Autodesk Inventor part; units mm, degrees
ref_plane "YZ Plane" through (0, 0, 0) normal (1, 0, 0) x (0, 1, 0)
ref_plane "XZ Plane" through (0, 0, 0) normal (0, 1, 0) x (-1, 0, 0)
ref_plane "XY Plane" through (0, 0, 0) normal (0, 0, 1) x (1, 0, 0)
sketch "Sketch1" plane through (0, 0, 0) normal (0, 1, 0) x (-1, 0, 0)
  line L0 (0, 0) -> (0, -140)
  line L1 (0, -140) -> (40, -140)
  line L2 (40, -140) -> (40, 0)
  line L3 (40, 0) -> (0, 0)
  dimension "d0" = 140
  dimension "d1" = 40
extrude "Extrusion1" add sketch "Sketch1" along normal blind 68.5
sketch "Sketch2" plane through (0, 0, 0) normal (1, 0, 0) x (0, 0, -1)
  line L0 (140, 68.5) -> (0, 68.5)
  line L1 (45, 78.5) -> (39, 78.5)
  line L2 (39, 78.5) -> (39, 74.5)
  line L3 (39, 74.5) -> (37.3, 74.5)
  line L4 (37.3, 74.5) -> (37.3, 80.2)
  line L5 (37.3, 80.2) -> (43.5, 80.2)
  line L6 (43.5, 80.2) -> (43.5, 104.7)
  line L7 (43.5, 104.7) -> (37.3, 104.7)
  line L8 (37.3, 104.7) -> (37.3, 110.4)
  line L9 (37.3, 110.4) -> (39, 110.4)
  line L10 (39, 110.4) -> (39, 106.4)
  line L11 (39, 106.4) -> (45, 106.4)
  line L12 (45, 106.4) -> (45, 78.5)
  line L13 (95, 78.5) -> (101, 78.5)
  line L14 (101, 78.5) -> (101, 74.5)
  line L15 (101, 74.5) -> (102.7, 74.5)
  line L16 (102.7, 74.5) -> (102.7, 80.2)
  line L17 (102.7, 80.2) -> (96.5, 80.2)
  line L18 (96.5, 80.2) -> (96.5, 104.7)
  line L19 (96.5, 104.7) -> (102.7, 104.7)
  line L20 (102.7, 104.7) -> (102.7, 110.4)
  line L21 (102.7, 110.4) -> (101, 110.4)
  line L22 (101, 110.4) -> (101, 106.4)
  line L23 (101, 106.4) -> (95, 106.4)
  line L24 (95, 106.4) -> (95, 78.5)
  line L25 (37.3, 68.5) -> (32.3, 68.5)
  line L26 (32.3, 68.5) -> (32.3, 110.4)
  line L27 (32.3, 110.4) -> (32.3, 115.4)
  line L28 (32.3, 115.4) -> (102.7, 115.4)
  line L29 (102.7, 115.4) -> (107.7, 115.4)
  line L30 (107.7, 115.4) -> (107.7, 68.5)
  line L31 (37.3, 68.5) -> (107.7, 68.5)
  point P0 (0, 0)
  dimension "d8" = 4
  dimension "d9" = 1.7
  dimension "d10" = 5.7
  dimension "d11" = 6.2
  dimension "d12" = 24.5
  dimension "d13" = 5.7
  dimension "d14" = 1.7
  dimension "d15" = 4
  dimension "d16" = 6
  dimension "d17" = 5
  dimension "d18" = 5
  dimension "d19" = 5
extrude "Extrusion2" add sketch "Sketch2" against normal up to surface (40 mm away)
sketch "Sketch3" plane through (0, 0, 0) normal (1, 0, 0) x (0, 0, -1)
  line L0 (87.95, 12.7) -> (87.95, 11)
  line L1 (87.95, 11) -> (83.95, 11)
  line L2 (83.95, 11) -> (83.95, 5)
  line L3 (83.95, 5) -> (70, 5)
  line L4 (70, 6.5) -> (82.25, 6.5)
  line L5 (82.25, 6.5) -> (82.25, 12.7)
  line L6 (82.25, 12.7) -> (87.95, 12.7)
  line L7 (52.05, 12.7) -> (52.05, 11)
  line L8 (52.05, 11) -> (56.05, 11)
  line L9 (56.05, 11) -> (56.05, 5)
  line L10 (56.05, 5) -> (70, 5)
  line L11 (70, 6.5) -> (57.75, 6.5)
  line L12 (57.75, 6.5) -> (57.75, 12.7)
  line L13 (57.75, 12.7) -> (52.05, 12.7)
  line L14 (107.7, 115.4) -> (32.3, 115.4)
  line L15 (87.95, 110.4) -> (87.95, 108.7)
  line L16 (87.95, 108.7) -> (83.95, 108.7)
  line L17 (83.95, 108.7) -> (83.95, 102.7)
  line L18 (83.95, 102.7) -> (70, 102.7)
  line L19 (70, 104.2) -> (82.25, 104.2)
  line L20 (82.25, 110.4) -> (87.95, 110.4)
  line L21 (52.05, 110.4) -> (52.05, 108.7)
  line L22 (52.05, 108.7) -> (56.05, 108.7)
  line L23 (56.05, 108.7) -> (56.05, 102.7)
  line L24 (56.05, 102.7) -> (70, 102.7)
  line L25 (70, 104.2) -> (57.75, 104.2)
  line L26 (57.75, 104.2) -> (57.75, 110.4)
  line L27 (57.75, 110.4) -> (52.05, 110.4)
  line L28 (82.25, 104.2) -> (82.25, 110.4)
  line L29 (140, 0) -> (0, 0)
  dimension "d27" = 6
  dimension "d31" = 6
extrude "Extrusion3" cut sketch "Sketch3" against normal up to surface (40 mm away)
sketch "Sketch4" plane through (0, 115.4, -32.3) normal (0, 1, 0) x (1, 0, 0)
  line L0 (-40, 75.4) -> (-40, 0)
  line L1 (0, 0) -> (-40, 0)
  line L2 (0, 75.4) -> (0, 0)
  line L3 (0, 75.4) -> (-40, 75.4)
  line L4 (0, -32.3) -> (0, 107.7)
  line L5 (-40, 107.7) -> (-40, -32.3)
  line L6 (-40, 75.4) -> (0, 75.4)
  line L7 (0, 0) -> (-40, 0)
  circle A0 centre (-30, 37.7) radius 3.05
  circle A1 centre (-10, 37.7) radius 3.05
  dimension "d48" = 6.1
  dimension "d49" = 6.1
sketch "Sketch5" plane through (0, 68.5, -107.7) normal (0, 0, -1) x (-1, 0, 0)
  line L0 (40, 0) -> (40, 46.9)
  line L1 (0, 46.9) -> (40, 46.9)
  line L2 (0, 0) -> (0, 46.9)
  line L3 (40, 0) -> (0, 0)
  line L4 (0, 46.9) -> (0, 0)
  line L5 (40, 36.2) -> (40, 11.7)
  line L6 (0, 46.9) -> (40, 46.9)
  circle A0 centre (20, 23.45) radius 3.05
  point P0 (0, -68.5)
sketch "Sketch6" plane through (0, 68.5, 0) normal (0, 1, 0) x (1, 0, 0)
  line L0 (-40, 107.7) -> (0, 107.7)
  line L1 (0, 107.7) -> (0, 140)
  line L2 (0, 140) -> (-40, 140)
  line L3 (-40, 140) -> (-40, 107.7)
  line L4 (0, 32.3) -> (-40, 32.3)
  line L5 (-40, 32.3) -> (-40, 0)
  line L6 (-40, 0) -> (0, 0)
  line L7 (0, 0) -> (0, 32.3)
  line L8 (0, 107.7) -> (0, 140)
  line L9 (-40, 140) -> (-40, 107.7)
  line L10 (0, 140) -> (-40, 140)
  line L11 (0, 32.3) -> (-40, 32.3)
  line L12 (-40, 0) -> (0, 0)
  line L13 (0, 0) -> (0, 140)
  line L14 (-40, 140) -> (-40, 0)
  circle A0 centre (-10, 123.85) radius 3.05
  circle A1 centre (-30, 123.85) radius 3.05
  circle A2 centre (-10, 16.15) radius 3.05
  circle A3 centre (-30, 16.15) radius 3.05
  dimension "d37" = 6.1
  dimension "d38" = 6.1
  dimension "d39" = 6.1
  dimension "d40" = 6.1
extrude "Extrusion4" cut sketch "Sketch6" against normal up to surface (68.5 mm away) contours A0 | A1 | A2 | A3
extrude "Extrusion5" cut sketch "Sketch4" against normal up to surface (115.4 mm away) contours A0 | A1
extrude "Extrusion6" cut sketch "Sketch5" against normal up to surface (75.4 mm away) contours A0
sketch "Sketch7" plane through (0, 0, 0) normal (1, 0, 0) x (0, 0, -1)
  line L0 (107.7, 53.5) -> (107.7, 23.5)
  line L1 (107.7, 23.5) -> (32.3, 23.5)
  line L2 (32.3, 23.5) -> (32.3, 53.5)
  line L3 (70, 23.5) -> (64, 23.5)
  line L4 (64, 23.5) -> (76, 23.5)
  line L5 (58, 53.5) -> (58, 93.5)
  line L6 (58, 93.5) -> (76, 93.5)
  line L7 (76, 93.5) -> (82, 93.5)
  line L8 (82, 93.5) -> (82, 53.5)
  line L9 (32.3, 53.5) -> (58, 53.5)
  line L10 (82, 53.5) -> (107.7, 53.5)
  line L11 (82, 93.5) -> (82, 83.5)
  line L12 (82, 83.5) -> (58, 83.5)
  point P0 (0, 0)
  dimension "d52" = 6
  dimension "d53" = 12
  dimension "d58" = 40
  dimension "d59" = 6
  dimension "d61" = 10
extrude "Extrusion7" cut sketch "Sketch7" against normal up to surface (40 mm away) contours L0 L1 L2 L9 L5 L12 L8 L10
fillet "Fillet1" radius 5 8 edges at (-20, 53.5, -82) (-20, 53.5, -58) (-20, 53.5, -32.3) (-20, 23.5, -32.3) (-20, 23.5, -107.7) (-20, 53.5, -107.7) (-20, 83.5, -58) (-20, 83.5, -82)
fillet "Fillet2" radius 5 4 edges at (-20, 115.4, -32.3) (-20, 68.5, -32.3) (-20, 115.4, -107.7) (-20, 68.5, -107.7)
properties part number "din_damper_connector"
Geometry: final body of the model. Coordinates: model frame, mm. A direction names the side the tool comes from. Coordinates: 2 decimals unless noted, no trailing zeros. Order: outer loops, then holes, each group sorted by start corner. A loop starts at its lowest first (then second) coordinate and runs counter-clockwise, first axis right, second up.
Item 1: Section query A-A (y = 41.5). Output: boundary loops of the cut face in (x, z).
Answer:
outline: (-40, -140) - (0, -140) - (0, -107.7) - (-40, -107.7) - close; (-40, -32.3) - (0, -32.3) - (0, 0) - (-40, 0) - close; hole circle Ø6.1 at (-30, -123.85); hole circle Ø6.1 at (-30, -16.15); hole circle Ø6.1 at (-10, -123.85); hole circle Ø6.1 at (-10, -16.15)
Item 2: Section query D-D (x = -10). State how many separate pieces and enclosed holes the cut face has, then the cut area to 3 significant figures.
Answer:
separate pieces: 4
enclosed holes: 2
area: 8,700 mm2
Item 3: Section query B-B (y = 91.95). Output: boundary loops of the cut face in (x, z).
Answer:
outline: (-40, -107.7) - (-23.05, -107.7) - (-23.05, -96.5) - (-40, -96.5) - close; (-40, -95) - (-23.05, -95) - (-23.05, -45) - (-40, -45) - close; (-40, -43.5) - (-23.05, -43.5) - (-23.05, -32.3) - (-40, -32.3) - close; (-16.95, -107.7) - (0, -107.7) - (0, -96.5) - (-16.95, -96.5) - close; (-16.95, -95) - (0, -95) - (0, -45) - (-16.95, -45) - close; (-16.95, -43.5) - (0, -43.5) - (0, -32.3) - (-16.95, -32.3) - close; hole circle Ø6.1 at (-30, -70); hole circle Ø6.1 at (-10, -70)
Item 4: Access query for faces 3 (the face through (-20, 12.7, -55)), 4 (the face through (-20.28, 70, -30.87)). Directions: +Z, -Z, +X, -X, +Y, -Y. A direction counts if a zero-diameter tool reaches every point of the face in a straight line with its end or side. Return the directions, or none.
Answer:
face 3: +X, -X
face 4: +Z, +X, -X, +Y
Item 5: Material intervals for line 1 along Z through (x, y) = (-23.5, 100.5); line 2 along Z through (x, y) = (-2, 9.5); line 3 along Y through (x, z) = (-20, -70), sorted ascending.
Answer:
line 1: z = -107.7 to -96.5, -95 to -45, -43.5 to -32.3
line 2: z = -140 to -83.95, -82.25 to -57.75, -56.05 to 0
line 3: y = 0 to 5, 6.5 to 23.5, 83.5 to 88.9, 95 to 102.7, 104.2 to 115.4
Item 6: Section query C-C (z = -16.15). Output: boundary loops of the cut face in (x, y), then the cut area to 3 significant figures.
Answer:
outline: (-40, 0) - (-33.05, 0) - (-33.05, 68.5) - (-40, 68.5) - close; (-26.95, 0) - (-13.05, 0) - (-13.05, 68.5) - (-26.95, 68.5) - close; (-6.95, 0) - (0, 0) - (0, 68.5) - (-6.95, 68.5) - close
area: 1,900 mm2
Item 7: Contact query for flat-ended pins moving along their axis: P1, Ø8, axis at x = -28.5, y = 80, coming from the +Z side; P2, Ø1, axis at x = -10, z = -82, coming from the -Y side; P3, Ø3.5, axis at x = -30, z = -70, coming from the +Y side; P4, Ø1, axis at x = -9, y = 72, coming from the +Z side. Output: stop coordinate, or through.
Answer:
P1: stops at z = -32.3
P2: stops at y = 0
P3: passes through
P4: stops at z = -31.88
Item 8: Draft query along X for faces 1 (the face through (-20, 77, -102.7)), 2 (the face through (-27.1, 34.7, -124.8)). Return one class per face: released by +X, released by -X, zero draft, split by the parting line, or undercut.
Answer:
face 1: zero draft
face 2: undercut
